Build history of the part. All positions in model axes, mm. A direction names the side the tool comes from. Give positions to 0.01 mm unless a question says otherwise; leave off trailing zeros. Loops run counter-clockwise (first coordinate to the right, second up) from the corner with the lowest first, then second, coordinate; pieces in that order, holes last.
1) Flat gauge pins, fed straight in: P1, Ø10, axis at x = 38.5, y = -4.5, coming from the +Z side; P2, Ø8, axis at y = -23.5, z = 12.5, coming from the +X side; P3, Ø7, axis at y = -13.5, z = 11.5, coming from the +X side; P4, Ø6.5, axis at y = 1, z = 10, coming from the +X side. Where does each tip first touch, or does it go through?
2) Band-saw the part on A-A on z = 19.25. List the corners of the cut face in (x, y), then the cut area to 3 significant figures.
3) Wall check: line 1 (Y direction, x = -11.5, z = 7.5); line 2 (Y direction, x = -37, z = 11.5); line 3 (X direction, y = -17.5, z = 21.5). Give the ranges that are in metal, low to high.
4) Band-saw the part on C-C on y = -28.5. List the corners of the cut face in (x, z).
5) Two-plate mould, pull along X, no slides. Class faces 4 (the flat face through (-48.535, -13, 12)), 5 (the cylindrical face through (50.36, -14.35, 12.32)), 6 (the flat face through (-46, -19.307, 12)), 7 (the flat face through (-32, -38.799, 12)): +X half, -X half, draft (parallel to the pull), parting line (faces both ways), or undercut.
6) 3-axis set-ups, long thin cutter, end or side, ignore diameter. For faces 1 (the flat face through (-15.306, -38, 12)), 2 (the flat face through (1, -36, 0)), 3 (the flat face through (-10, -35.799, 12)): which of +Z, -Z, +X, -X, +Y, -Y reach the whole face in a straight line?
7) Band-saw the part on B-B on x = -41.5. List the corners of the cut face in (y, z), then the cut area to 3 significant figures.
```python
from build123d import *

# Parameters (mm, degrees)
F1_DEPTH = 25


with BuildPart() as f1:
    # F0 (on Top) → F1 (new body)
    with BuildSketch(Plane.XY):
        with BuildLine():
            Line((-30.05274, 11.200704), (-48.534881, 11.200704))
            Line((-48.534881, 11.200704), (-48.534881, -38.799296))
            Line((-48.534881, -38.799296), (-15.306122, -38.799296))
            Line((-15.306122, -38.799296), (-15.306122, -36.599296))
            Line((-15.306122, -36.599296), (-6.91196, -36.599296))
            Line((-6.91196, -36.599296), (-6.91196, -38.799296))
            Line((-6.91196, -38.799296), (25.364829, -38.799296))
            ThreePointArc((25.364829, -38.799296), (50.364829, -13.799296), (25.364829, 11.200704))
            Line((25.364829, 11.200704), (-19.365611, 11.200704))
            Line((-19.365611, 11.200704), (-30.05274, 11.200704))
        make_face()
        with BuildLine():
            Line((-45.534881, -5.245955), (-45.534881, 8.200704))
            Line((-45.534881, 8.200704), (-34.456972, 8.200704))
            Line((-34.456972, 8.200704), (-34.456972, 10.400704))
            Line((-34.456972, 10.400704), (-20.740092, 10.400704))
            Line((-20.740092, 10.400704), (-20.740092, 8.200704))
            Line((-20.740092, 8.200704), (25.364829, 8.200704))
            ThreePointArc((25.364829, 8.200704), (47.364829, -13.799296), (25.364829, -35.799296))
            Line((25.364829, -35.799296), (-45.534881, -35.799296))
            Line((-45.534881, -35.799296), (-45.534881, -19.307144))
            Line((-45.534881, -19.307144), (-47.334881, -19.307144))
            Line((-47.334881, -19.307144), (-47.334881, -5.245955))
            Line((-47.334881, -5.245955), (-45.534881, -5.245955))
        make_face(mode=Mode.SUBTRACT)
    extrude(amount=F1_DEPTH)


solid = f1.part
```
Findings below:
1. P1: passes through
1. P2: stops at x = 49.71
1. P3: stops at x = 50.36
1. P4: stops at x = 47.54
2. outline: (-48.53, -38.8) - (-15.31, -38.8) - (-15.31, -36.6) - (-6.91, -36.6) - (-6.91, -38.8) - (25.36, -38.8) arc R25 ccw to (25.36, 11.2) - (-48.53, 11.2) - close; hole (-47.33, -19.31) - (-45.53, -19.31) - (-45.53, -35.8) - (25.36, -35.8) arc R22 ccw to (25.36, 8.2) - (-20.74, 8.2) - (-20.74, 10.4) - (-34.46, 10.4) - (-34.46, 8.2) - (-45.53, 8.2) - (-45.53, -5.25) - (-47.33, -5.25) - close
2. area: 723 mm2
3. line 1: y = -36.6 to -35.8, 8.2 to 11.2
3. line 2: y = -38.8 to -35.8, 8.2 to 11.2
3. line 3: x = -48.53 to -47.33, 47.05 to 50.09
4. outline: (-48.53, 0) - (-45.53, 0) - (-45.53, 25) - (-48.53, 25) - close; (41.73, 0) - (45.59, 0) - (45.59, 25) - (41.73, 25) - close
5. face 4: -X half
5. face 5: +X half
5. face 6: undercut
5. face 7: draft
6. face 1: +Z, -Z, -Y
6. face 2: -Z, +X, -X, +Y, -Y
6. face 3: +Z, -Z
7. outline: (-38.8, 0) - (-35.8, 0) - (-35.8, 25) - (-38.8, 25) - close; (8.2, 0) - (11.2, 0) - (11.2, 25) - (8.2, 25) - close
7. area: 150 mm2
